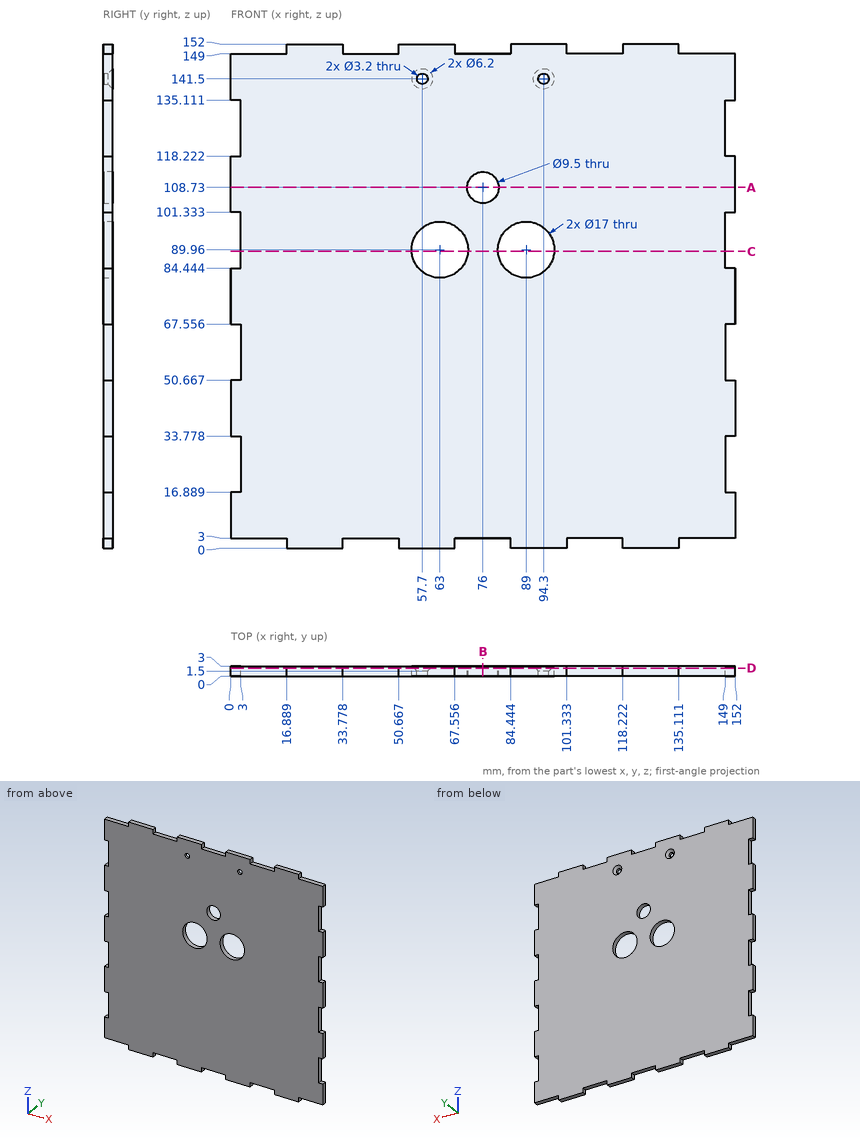
Input: dimensioned drawing with shaded views. Units: mm. Origin: part minimum x, y, z. Round coordinates to 2 decimals unless told otherwise and drop trailing zeros. Loops run counter-clockwise (first coordinate to the right, second up) from the corner with the lowest first, then second, coordinate; pieces in that order, holes last. Notation, with made-up numbers: (68, 15.5) -> (95, 15.5) arc R23 cw to (95, 39.5) -> close; hole circle Ø1 at (83.5, -17). An arc over 180 degrees is marked (long way). Answer as a JSON object with one key per item and string values. Group by question number.
1) Pin query (flat end, axial travel): pin 1 (1.5 mm diameter, centred on x = 1.5, y = 1.5, fed in from +Z); pin 2 (0.9 mm diameter, centred on x = 151, y = 1.5, fed in from -Z); pin 3 (0.9 mm diameter, centred on y = 1.5, z = 62, fed in from -X). Return the tip coordinate at first contact, or that it passes through.
2) Section query B-B on x = 76. Output: boundary loops of the cut face in (y, z).
3) Section query D-D on y = 2.4. State how many separate pieces and enclosed holes the cut face has, plus the area to 3 significant figures.
4) Section query A-A on z = 108.73. Output: boundary loops of the cut face in (x, y).
5) Ray query, L1, parallel to X at y = 2.15, z = 89.96; L2, parallel to X at y = 0.7, z = 141.5; L3, parallel to X at y = 2.45, z = 108.73. Return the intervals inside material, ascending.
6) Section query C-C on z = 89.5. Output: boundary loops of the cut face in (x, y).
Reply:
{
 "1": {"pin 1": "stops at z = 149", "pin 2": "stops at z = 3", "pin 3": "stops at x = 3"},
 "2": {"outline": "(0, 3) -> (3, 3) -> (3, 103.98) -> (0, 103.98) -> close; (0, 113.48) -> (3, 113.48) -> (3, 149) -> (0, 149) -> close"},
 "3": {"separate pieces": "1", "enclosed holes": "5", "area": "21,600 mm2"},
 "4": {"outline": "(0, 0) -> (71.25, 0) -> (71.25, 3) -> (0, 3) -> close; (80.75, 0) -> (152, 0) -> (152, 3) -> (80.75, 3) -> close"},
 "5": {"L1": "x = 3 to 54.5, 71.5 to 80.5, 97.5 to 149", "L2": "x = 0 to 56.1, 59.3 to 92.7, 95.9 to 152", "L3": "x = 0 to 71.25, 80.75 to 152"},
 "6": {"outline": "(3, 0) -> (54.51, 0) -> (54.51, 3) -> (3, 3) -> close; (71.49, 0) -> (80.51, 0) -> (80.51, 3) -> (71.49, 3) -> close; (97.49, 0) -> (149, 0) -> (149, 3) -> (97.49, 3) -> close"}
}
